Can you work these out from the model? Positions are in its coordinate system, mm. A direction names the side the tool comes from. Give positions to 0.01 mm unless a question says otherwise; leave off trailing zeros. Order: outer loops, then holes, each group sorted by start corner. A loop starts at its lowest first (then second) coordinate and runs counter-clockwise, first axis right, second up. Notation, with made-up numbers: (-11, -27.5) - (31, -27.5) arc R34 cw to (31, 4.5) - close; hole circle Ø5 at (-40, 39). An arc over 180 degrees is marked (long way). Use one line per item in the form item = value. Start each with the question number.
1) We'd pull the mould along X, two halves only. Please class faces 4 (the conical face through (-0.81, -0.01, 3.69)), 5 (the conical face through (-0.81, -3.19, -1.85)), 6 (the conical face through (-3.424, 3.149, -1.808)), 7 (the flat face through (-2.12, -1.726, -3.045)): released by +X, released by -X, zero draft, split by the parting line, or undercut.
2) Suppose I cut it at A-A, the plane x = 25. Write out the boundary of the cut face in (y, z), and give its area (3 significant figures).
3) Please list where these lines run through material, in increasing order: probe 1 along Y at (x, z) = (18, 0); probe 2 along X at (y, z) = (-2.5, -2.75); probe 3 along X at (y, z) = (1.5, 3).
4) For pin 1 (4 mm diameter, centred on x = 14.5, z = 3, fed in from -Y); pin 2 (3 mm diameter, centred on x = 24.5, y = 1, fed in from +Z); pin 3 (2 mm diameter, centred on x = -2.5, z = 0.5, fed in from +Y), each with a flat end and sliding along its axis, tell me the tip position at first contact or that it passes through.
5) Which directions (+Z, -Z, +X, -X, +Y, -Y) give clear straight access to the entire face, cutting with the end or side of a thin tool? Please do faces 1 (the conical face through (-0.81, 3.19, 1.85)), 2 (the flat face through (-2, 3.5, 0)), 3 (the flat face through (-2.1, -1.8, 3)).
```python
from build123d import *

# Parameters (mm, degrees)
SKETCH2_W          = 20
SKETCH2_H          = 20
CUT_EXTRUDE1_DEPTH = 5
SKETCH4_W          = 0.5
SKETCH4_H          = 1.75


with BuildPart() as part:
    # Sketch1 → Revolve1 (revolve)
    with BuildSketch(Plane.XY):
        with BuildLine():
            Line((-3.5, 0), (-3.5, 3.5))
            Line((-3.5, 3.5), (-2.1, 5.924871131))
            Line((-2.1, 5.924871131), (-0.7, 3.5))
            Line((-0.7, 3.5), (0, 3.5))
            Line((0, 3.5), (0, 2.5))
            Line((0, 2.5), (0.258578644, 2.241421356))
            ThreePointArc((0.258578644, 2.241421356), (0.4, 2.182842712), (0.541421356, 2.241421356))
            Line((0.541421356, 2.241421356), (0.8, 2.5))
            Line((0.8, 2.5), (3.7, 2.5))
            Line((3.7, 2.5), (4.3, 1.9))
            Line((4.3, 1.9), (4.3, 1.7))
            Line((4.3, 1.7), (43.4, 1.7))
            ThreePointArc((43.4, 1.7), (43.470710678, 1.670710678), (43.5, 1.6))
            Line((43.5, 1.6), (43.5, 1.3))
            ThreePointArc((43.5, 1.3), (43.529289322, 1.229289322), (43.6, 1.2))
            Line((43.6, 1.2), (44.8, 1.2))
            ThreePointArc((44.8, 1.2), (44.870710678, 1.229289322), (44.9, 1.3))
            Line((44.9, 1.3), (44.9, 1.6))
            ThreePointArc((44.9, 1.6), (44.929289322, 1.670710678), (45, 1.7))
            Line((45, 1.7), (45.566987298, 1.7))
            Line((45.566987298, 1.7), (46, 1.45))
            Line((46, 1.45), (46, 0))
            Line((46, 0), (-3.5, 0))
        make_face()
    revolve(axis=Axis((46, 0, 0), (-1, 0, 0)))

    # Sketch2 → Cut-Extrude1 (cut)
    with BuildSketch(Plane.ZY.offset(3.5)):
        Rectangle(SKETCH2_W, SKETCH2_H)
        Polygon((2.020725942, -3.5), (4.041451884, 0), (2.020725942, 3.5), (-2.020725942, 3.5), (-4.041451884, 0), (-2.020725942, -3.5), align=None, mode=Mode.SUBTRACT)
    extrude(amount=-CUT_EXTRUDE1_DEPTH, mode=Mode.SUBTRACT)

    # Sketch3 → Revolve2 (revolve)
    with BuildSketch(Plane.XY):
        with BuildLine():
            Line((43.5, 1.2), (44.9, 1.2))
            ThreePointArc((44.9, 1.2), (44.2, 1.9), (43.5, 1.2))
        make_face()
    revolve(axis=Axis((44.9, 0, 0), (-1, 0, 0)))

    # Sketch4 → Revolve3 (revolve)
    with BuildSketch(Plane.XY):
        with Locations((0.25, 3.025)):
            Rectangle(SKETCH4_W, SKETCH4_H)
    revolve(axis=Axis((0.5, 0, 0), (-1, 0, 0)))


solid = part.part
```
Result sheet:
q1.face_4 = undercut
q1.face_5 = undercut
q1.face_6 = released by -X
q1.face_7 = zero draft
q2.outline = circle Ø3.4 at (0, 0)
q2.area = 9.08 mm²
q3.probe_1 = -1.7 to 1.7
q3.probe_2 = 0 to 0.5
q3.probe_3 = -3.5 to 0.5
q4.pin_1 = -1.37
q4.pin_2 = 1.7
q4.pin_3 = 3.5
q5.face_1 = +Z, +Y
q5.face_2 = +Z, -Z, -X, +Y
q5.face_3 = +Z, -X, -Y
